from build123d import *

# Parameters (mm, degrees)
BOSS_EXTRUDE1_DEPTH = 0.3


with BuildPart() as part:
    # Sketch3 → Boss-Extrude1 (new body, symmetric)
    with BuildSketch(Plane.XY):
        with BuildLine():
            Line((0, 0), (-0.3, 0))
            Line((-0.3, 0), (-0.3, 6.4))
            ThreePointArc((-0.3, 6.4), (-0.124264069, 6.824264069), (0.3, 7))
            Line((0.3, 7), (7.3, 7))
            Line((7.3, 7), (7.3, 6.4))
            Line((7.3, 6.4), (0.5, 6.4))
            ThreePointArc((0.5, 6.4), (0.358578644, 6.341421356), (0.3, 6.2))
            Line((0.3, 6.2), (0.3, 0))
            Line((0.3, 0), (0, 0))
        make_face()
    extrude(amount=BOSS_EXTRUDE1_DEPTH, both=True)


solid = part.part
For this review, take the finished solid that the model builds, in its own axes (mm). Round coordinates to 2 decimals unless told otherwise and drop trailing zeros. Loops run counter-clockwise (first coordinate to the right, second up) from the corner with the lowest first, then second, coordinate; pieces in that order, holes last. Notation, with made-up numbers: (70.5, 60.5) - (123.5, 60.5) arc R33 ccw to (123.5, 99.5) - close; hole circle Ø1 at (24.25, -26.5). An arc over 180 degrees is marked (long way). Use one line per item in the form item = value.
1) We need section B-B on y = 4.5. Write out the cut boundary in (x, z), then the cut area to 3 significant figures.
Solutions:
outline = (-0.3, -0.3) - (0.3, -0.3) - (0.3, 0.3) - (-0.3, 0.3) - close
area = 0.360 mm2
2) Wall thickness on probe 1 along Y at (x, z) = (4.25, 0.05); probe 2 along X at (y, z) = (3.5, 0); probe 3 along Y at (x, z) = (0.25, 0.05): over which ranges is each line inside the solid? List them lowest first.
Solutions:
probe_1 = 6.4 to 7
probe_2 = -0.3 to 0.3
probe_3 = 0 to 7
3) We need section C-C on x = 6.25. Write out the cut boundary in (y, z).
Solutions:
outline = (6.4, -0.3) - (7, -0.3) - (7, 0.3) - (6.4, 0.3) - close
4) We need section A-A on z = 0.1. Write out the cut boundary in (x, y), then the cut area to 3 significant figures.
Solutions:
outline = (-0.3, 0) - (0.3, 0) - (0.3, 6.2) arc R0.2 cw to (0.5, 6.4) - (7.3, 6.4) - (7.3, 7) - (0.3, 7) arc R0.6 ccw to (-0.3, 6.4) - close
area = 8.33 mm2
